Autodesk Inventor part; units mm, degrees
ref_plane "YZ Plane" through (0, 0, 0) normal (1, 0, 0) x (0, 1, 0)
ref_plane "XZ Plane" through (0, 0, 0) normal (0, 1, 0) x (-1, 0, 0)
sketch "Sketch1" plane through (0, 0, 0) normal (0, 0, 1) x (1, 0, 0)
  line L0 (0, 0) -> (135, 0) construction
  line L1 (135, 0) -> (270, 0) construction
  circle A0 centre (0, 0) radius 10
  circle A1 centre (270, 0) radius 10
  circle A2 centre (0, 0) radius 20
  circle A3 centre (270, 0) radius 20
  line L2 (0, 20) -> (270, 20)
  line L3 (0, -20) -> (270, -20)
  circle A4 centre (135, 0) radius 10
  dimension "d0" = 135
  dimension "d1" = 20
  dimension "d2" = 20
  dimension "d3" = 40
  dimension "d4" = 40
  dimension "d7" = 20
extrude "Extrusion1" add sketch "Sketch1" along normal blind 10
ref_plane "Work Plane1" through (0, 0, 5) normal (0, 0, 1) x (1, 0, 0)
properties part number "EslabonPreliminarElevacion"
Input: part model. Units: mm. Frame: model coordinates. Coordinates: 2 decimals unless noted, no trailing zeros. Loops run counter-clockwise (first coordinate to the right, second up) from the corner with the lowest first, then second, coordinate; pieces in that order, holes last. Notation, with made-up numbers: (-0.5, 15.5) -> (41.5, 15.5) arc R38 cw to (41.5, 53.5) -> close; hole circle Ø3 at (31.25, 89.5). An arc over 180 degrees is marked (long way). Write each question's results on one line, items separated by ' | '. Start each with the question number.
Q1. Section C-C, the plane z = 7. Return the cut outline in (x, y).
Q2. Ray query, line 1 (X direction, y = -1, z = 6); line 2 (Y direction, x = 270, z = 6.75); line 3 (X direction, y = -1.5, z = 8.5). Return the intervals inside material, ascending. Write a range as from..to.
Q3. Section A-A, the plane y = 0. Return the cut outline in (x, z).
Q4. Section B-B, the plane x = 135. Return the cut outline in (y, z), plus the area to 3 significant figures.
Q5. Section D-D, the plane y = -13. Return the cut outline in (x, z).
Q6. Pin query (flat end, axial travel): pin 1 (5 mm diameter, centred on x = 199, y = 14.5, fed in from -Z); pin 2 (16 mm diameter, centred on x = 135, y = 0, fed in from +Z); pin 3 (1.5 mm diameter, centred on y = -4, z = 6, fed in from -X); pin 4 (3 mm diameter, centred on y = -5.5, z = 5, fed in from +X). Return the tip coordinate at first contact, or that it passes through.
Q7. Pull-direction query (X, two-part tool) for faces 1 (the cylindrical face through (144.237, 3.83, 4.93)), 2 (the flat face through (133, -20, 5)), 3 (the cylindrical face through (-20, 0, 5)); classes: released by +X, released by -X, zero draft, split by the parting line, or undercut.
Found:
1) outline: (0, -20) -> (270, -20) arc R20 ccw to (270, 20) -> (0, 20) arc R20 ccw to start; hole circle Ø20 at (0, 0); hole circle Ø20 at (135, 0); hole circle Ø20 at (270, 0)
2) line 1: -19.97..-9.95, 9.95..125.05, 144.95..260.05, 279.95..289.97 | line 2: -20..-10, 10..20 | line 3: -19.94..-9.89, 9.89..125.11, 144.89..260.11, 279.89..289.94
3) outline: (-20, 0) -> (-10, 0) -> (-10, 10) -> (-20, 10) -> close; (10, 0) -> (125, 0) -> (125, 10) -> (10, 10) -> close; (145, 0) -> (260, 0) -> (260, 10) -> (145, 10) -> close; (280, 0) -> (290, 0) -> (290, 10) -> (280, 10) -> close
4) outline: (-20, 0) -> (-10, 0) -> (-10, 10) -> (-20, 10) -> close; (10, 0) -> (20, 0) -> (20, 10) -> (10, 10) -> close | area: 200 mm2
5) outline: (-15.2, 0) -> (285.2, 0) -> (285.2, 10) -> (-15.2, 10) -> close
6) pin 1: z = 0 | pin 2: through | pin 3: x = -19.73 | pin 4: x = 289.6
7) face 1: undercut | face 2: zero draft | face 3: released by -X
